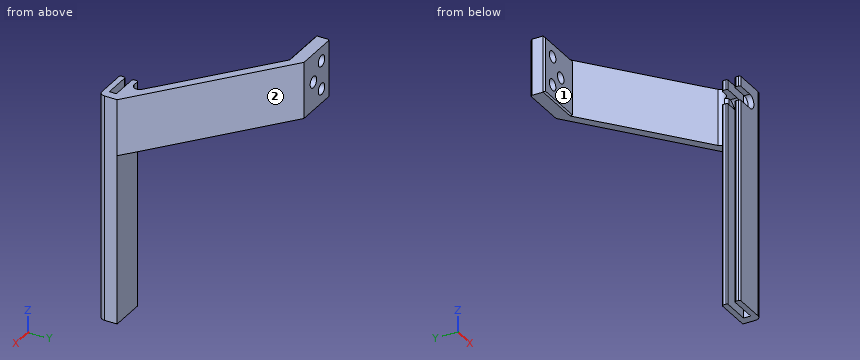
```python
from build123d import *

# Parameters (mm, degrees)
EXTRUDE_1_DEPTH     = 20
SKETCH_2_R          = 2.5
SKETCH_2_W          = 0.5
SKETCH_2_H          = 5
CUT_EXTRUDE_1_DEPTH = 7
FILLET_2_R          = 1
EXTRUDE_START       = 60
EXTRUDE_2_DEPTH     = 60
SKETCH_4_R          = 2
CUT_EXTRUDE_2_DEPTH = 5
CHAMFER_1_SIZE      = 0.5


with BuildPart() as part:
    # 草图1 → 凸台-拉伸1 (new body)
    with BuildSketch(Plane.XY):
        with BuildLine():
            Line((51.5, 0), (62, 0))
            ThreePointArc((62, 0), (63.414213562, 0.585786438), (64, 2))
            Line((64, 2), (64, 6.5))
            Line((64, 6.5), (15.818440015, 45))
            Line((15.818440015, 45), (0, 45))
            Line((0, 45), (0, 40))
            Line((0, 40), (17.27, 40))
            Line((17.27, 40), (54.735914555, 10.062453129))
            ThreePointArc((54.735914555, 10.062453129), (55.374865565, 7.838526742), (53.487419373, 6.5))
            Line((53.487419373, 6.5), (51.5, 6.5))
            ThreePointArc((51.5, 6.5), (51.146446609, 6.353553391), (51, 6))
            Line((51, 6), (51, 5))
            ThreePointArc((51, 5), (51.146446609, 4.646446609), (51.5, 4.5))
            Line((51.5, 4.5), (61, 4.5))
            Line((61, 4.5), (61, 2))
            Line((61, 2), (51.5, 2))
            ThreePointArc((51.5, 2), (51.146446609, 1.853553391), (51, 1.5))
            Line((51, 1.5), (51, 0.5))
            ThreePointArc((51, 0.5), (51.146446609, 0.146446609), (51.5, 0))
        make_face()
    extrude(amount=EXTRUDE_1_DEPTH)

    # 草图2 → 切除-拉伸1 (cut)
    with BuildSketch(Plane.XZ):
        with Locations((57, 14)):
            Circle(SKETCH_2_R)
        with BuildLine():
            Line((57, 16.5), (51.5, 16.5))
            Line((51.5, 16.5), (51.5, 11.5))
            Line((51.5, 11.5), (57, 11.5))
            ThreePointArc((57, 11.5), (54.5, 14), (57, 16.5))
        make_face()
        with Locations((51.25, 14)):
            Rectangle(SKETCH_2_W, SKETCH_2_H)
    extrude(amount=-CUT_EXTRUDE_1_DEPTH, mode=Mode.SUBTRACT)

    # 圆角2
    fillet_2_edges = [part.edges().sort_by_distance(p)[0] for p in [
        (54.810295028, 7, 14),
    ]]
    fillet(fillet_2_edges, radius=FILLET_2_R)

    # 草图3 → 凸台-拉伸2 (add)
    with BuildSketch(Plane(origin=(0, 0, 0), x_dir=(-1, 0, 0), z_dir=(0, 0, -1)).offset(EXTRUDE_START)):
        with BuildLine():
            Line((-64, 6.5), (-53.487419373, 6.5))
            Line((-53.487419373, 6.5), (-51.5, 6.5))
            ThreePointArc((-51.5, 6.5), (-51.146446609, 6.353553391), (-51, 6))
            Line((-51, 6), (-51, 5))
            ThreePointArc((-51, 5), (-51.146446609, 4.646446609), (-51.5, 4.5))
            Line((-51.5, 4.5), (-61, 4.5))
            Line((-61, 4.5), (-61, 2))
            Line((-61, 2), (-51.5, 2))
            ThreePointArc((-51.5, 2), (-51.146446609, 1.853553391), (-51, 1.5))
            Line((-51, 1.5), (-51, 0.5))
            ThreePointArc((-51, 0.5), (-51.146446609, 0.146446609), (-51.5, 0))
            Line((-51.5, 0), (-62, 0))
            ThreePointArc((-62, 0), (-63.414213562, 0.585786438), (-64, 2))
            Line((-64, 2), (-64, 6.5))
        make_face()
    extrude(amount=-EXTRUDE_2_DEPTH)

    # 草图4 → 切除-拉伸2 (cut)
    with BuildSketch(Plane(origin=(0, 45, 0), x_dir=(1, 0, 0), z_dir=(0, 1, 0))):
        with Locations(Location((5, -5, 0), (0, 0, 270))):
            Circle(SKETCH_4_R)
        with Locations(Location((5, -15, 0), (0, 0, 270))):
            Circle(SKETCH_4_R)
        with Locations(Location((10, -10, 0), (0, 0, 270))):
            Circle(SKETCH_4_R)
    extrude(amount=-CUT_EXTRUDE_2_DEPTH, mode=Mode.SUBTRACT)

    # 倒角1
    chamfer_1_edges = [part.edges().sort_by_distance(p)[0] for p in [
        (8.635, 40, 20),
        (8.635, 40, 0),
        (0, 40, 10),
        (0, 45, 10),
    ]]
    chamfer(chamfer_1_edges, length=CHAMFER_1_SIZE)


solid = part.part
```
Model file for the job. Use its own axes, mm. Face numbers are marked on the shaded views. A direction names the side the tool comes from. Give positions to 0.01 mm unless a question says otherwise; leave off trailing zeros. Write each loop counter-clockwise with the first axis right and the second up, starting at its lowest first coordinate (ties: lowest second). Pieces come first, ordered by that corner, then holes. Notation, with made-up numbers: (78.5, 69.25) - (85.5, 69.25) arc R16 ccw to (85.5, 86.25) - close; hole circle Ø6 at (36, -36). An arc over 180 degrees is marked (long way). One line per question, with ' | ' between items. Start each with the question number.
(1) Pin check, flat tips, straight feed: P1, Ø6, axis at x = 56, z = -37, coming from the +Y side; P2, Ø5, axis at x = 58.5, z = -0.5, coming from the -Y side; P3, Ø8, axis at x = 39.5, y = 30.5, coming from the -Z side; P4, Ø5, axis at x = 7, z = 8.5, coming from the -Y side. Stop position of each tip, or through.
(2) 3-axis set-ups, long thin cutter, end or side, ignore diameter. For the marked faces 1 and 2: which of +Z, -Z, +X, -X, +Y, -Y reach the whole face in a straight line?
(3) Slice it at D-D on z = 14. Write the cut outline in (x, y), plus the area to 3 significant figures.
(4) Slice it at A-A on x = 5. Write the cut outline in (y, z).
(5) Slice it at C-C on z = -19.5. Write the cut outline in (x, y).
(6) Wall check: line 1 along Y through (x, z) = (54, 3); line 2 along Y through (x, z) = (56, -6); line 3 along X through (y, z) = (43.5, 9.5). Give the ranges that are in metal, low to high. Write a range as from..to.
(7) Slice it at B-B on z = 5. Write the cut outline in (x, y).
Results below:
1) P1: y = 6.5 | P2: y = 0 | P3: z = 0 | P4: y = 40
2) face 1: +Z, -Z, -X, -Y | face 2: +Z, -Z, +X, +Y
3) outline: (0, 40.5) - (0.5, 40) - (3.27, 40) - (3.27, 45) - (0.5, 45) - (0, 44.5) - close; (6.73, 40) - (17.27, 40) - (54.74, 10.06) arc R2 cw to (55.46, 8.17) arc R1 ccw to (56.45, 7) - (59.5, 7) - (59.5, 4.5) - (61, 4.5) - (61, 2) - (59.5, 2) - (59.5, 0) - (62, 0) arc R2 ccw to (64, 2) - (64, 6.5) - (15.82, 45) - (6.73, 45) - close | area: 266 mm^2
4) outline: (40, 0.5) - (40.5, 0) - (45, 0) - (45, 3) - (40, 3) - close; (40, 7) - (45, 7) - (45, 13) - (40, 13) - close; (40, 17) - (45, 17) - (45, 20) - (40.5, 20) - (40, 19.5) - close
5) outline: (51, 0.5) arc R0.5 ccw to (51.5, 0) - (62, 0) arc R2 ccw to (64, 2) - (64, 6.5) - (51.5, 6.5) arc R0.5 ccw to (51, 6) - (51, 5) arc R0.5 ccw to (51.5, 4.5) - (61, 4.5) - (61, 2) - (51.5, 2) arc R0.5 ccw to (51, 1.5) - close
6) line 1: 0..2, 4.5..6.57, 10.65..14.49 | line 2: 0..2, 4.5..6.5 | line 3: 0..8.06, 11.94..17.7
7) outline: (0, 40.5) - (0.5, 40) - (3, 40) - (3, 45) - (0.5, 45) - (0, 44.5) - close; (7, 40) - (17.27, 40) - (54.74, 10.06) arc R2 cw to (53.49, 6.5) - (51.5, 6.5) arc R0.5 ccw to (51, 6) - (51, 5) arc R0.5 ccw to (51.5, 4.5) - (61, 4.5) - (61, 2) - (51.5, 2) arc R0.5 ccw to (51, 1.5) - (51, 0.5) arc R0.5 ccw to (51.5, 0) - (62, 0) arc R2 ccw to (64, 2) - (64, 6.5) - (15.82, 45) - (7, 45) - close
